from build123d import *

# Parameters (mm, degrees)
F0_W     = 50
F0_H     = 160
F0_W_2   = 10
F0_H_2   = 140
F1_DEPTH = 15
F2_DEPTH = 30
F3_R     = 3
F4_DEPTH = 25
F0_W_3   = 15
F5_DEPTH = 25


with BuildPart() as f1:
    # F0 (on Front) → F1 (new body)
    with BuildSketch(Plane.XZ):
        with Locations((0, 20)):
            Rectangle(F0_W, F0_H)
        with Locations((0, 15)):
            Rectangle(F0_W_2, F0_H_2, mode=Mode.SUBTRACT)
    extrude(amount=F1_DEPTH)

    # F0 (on Front) → F2 (join)
    with BuildSketch(Plane.XZ):
        Polygon((-40, -100), (40, -100), (40, -60), (25, -60), (-25, -60), (-40, -60), align=None)
    extrude(amount=F2_DEPTH)

    # F3 (on face) → F4 (cut)
    with BuildSketch(Plane(origin=(0, 0, -100), x_dir=(1, 0, 0), z_dir=(0, 0, -1))):
        with Locations((-10, 15)):
            Circle(F3_R)
        with Locations((10, 15)):
            Circle(F3_R)
    extrude(amount=-F4_DEPTH, mode=Mode.SUBTRACT)

    # F0 (on Front) → F5 (join)
    with BuildSketch(Plane.XZ):
        with Locations((-32.5, 20)):
            Rectangle(F0_W_3, F0_H)
        with Locations((32.5, 20)):
            Rectangle(F0_W_3, F0_H)
    extrude(amount=F5_DEPTH)


solid = f1.part
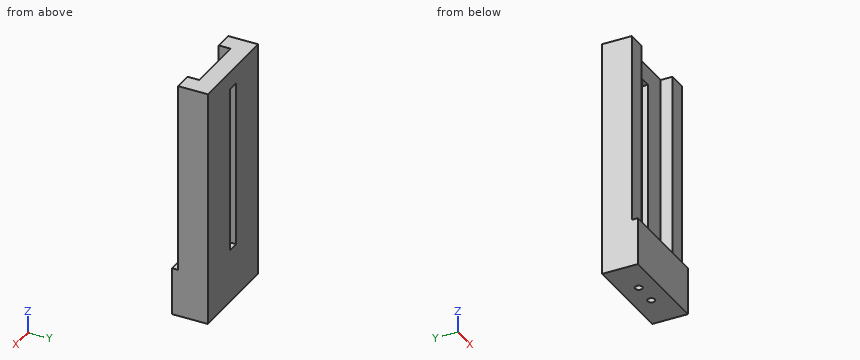
Check sheet for the modelled part. Datum: model origin and axes. Units: mm. Give positions to 0.01 mm unless a question says otherwise; leave off trailing zeros. Write each loop counter-clockwise with the first axis right and the second up, starting at its lowest first coordinate (ties: lowest second). Pieces come first, ordered by that corner, then holes. Notation, with made-up numbers: (82, 5) -> (104, 5) arc R30 cw to (104, 40) -> close; hole circle Ø2 at (49.25, -31). An arc over 180 degrees is marked (long way). Write item = value, one per line.
Item 1: Sectioned sample at A-A on z = -46. Record the boundary of the cut face in (x, y).
Output:
outline = (-40, -25) -> (-25, -25) -> (-25, -15) -> (-5, -15) -> (-5, 0) -> (-40, 0) -> close; (5, -15) -> (25, -15) -> (25, -25) -> (40, -25) -> (40, 0) -> (5, 0) -> close
Item 2: Scan lines: probe 1 along X at (y, z) = (-15, -89.5); probe 2 along X at (y, z) = (-23.5, 84.5); probe 3 along X at (y, z) = (-1.25, 54). Record each from-to range of solid material in increasing order. Write a range as from..to.
Output:
probe_1 = -40..-13, -7..7, 13..40
probe_2 = -40..-25, 25..40
probe_3 = -40..-5, 5..40
Item 3: Sectioned sample at C-C on y = -2.75. Record the boundary of the cut face in (x, z).
Output:
outline = (-40, -100) -> (40, -100) -> (40, 100) -> (-40, 100) -> close; hole (-5, -55) -> (5, -55) -> (5, 85) -> (-5, 85) -> close
Item 4: Gauge pin test, flat ends, axial feed: pin 1 (4 mm diameter, centred on x = 23.5, z = -71.5, fed in from +Y); pin 2 (1.8 mm diameter, centred on x = 11, y = -14.5, fed in from -Z); pin 3 (7.5 mm diameter, centred on x = 3.5, y = -22, fed in from +Z); pin 4 (6 mm diameter, centred on x = 25, z = 74.5, fed in from -Y). Record the tip position at first contact, or that the pin passes through.
Output:
pin_1 = 0
pin_2 = -75
pin_3 = -60
pin_4 = -25
Item 5: Sectioned sample at B-B on x = -1. Record the boundary of the cut face in (y, z), and give its area (3 significant figures).
Output:
outline = (-30, -100) -> (0, -100) -> (0, -55) -> (-15, -55) -> (-15, -60) -> (-30, -60) -> close; (-15, 85) -> (0, 85) -> (0, 100) -> (-15, 100) -> close
area = 1,500 mm^2
Item 6: Sectioned sample at D-D on z = -77.5. Record the boundary of the cut face in (x, y).
Output:
outline = (-40, -30) -> (40, -30) -> (40, 0) -> (-40, 0) -> close; hole circle Ø6 at (-10, -15); hole circle Ø6 at (10, -15)
